```python
from build123d import *

# Parameters (mm, degrees)
SKETCH1_W           = 220
SKETCH1_H           = 220
BOSS_EXTRUDE1_DEPTH = 3
SKETCH2_W           = 220
SKETCH2_H           = 220
SKETCH2_W_2         = 204
SKETCH2_H_2         = 204
BOSS_EXTRUDE3_DEPTH = 22
SKETCH3_R           = 1
CUT_EXTRUDE1_DEPTH  = 313.1297807


with BuildPart() as part:
    # Sketch1 → Boss-Extrude1 (new body)
    with BuildSketch(Plane.XY):
        with Locations((110, 110)):
            Rectangle(SKETCH1_W, SKETCH1_H)
    extrude(amount=BOSS_EXTRUDE1_DEPTH)

    # Sketch2 → Boss-Extrude3 (add)
    with BuildSketch(Plane.XY.offset(3)):
        with Locations((110, 110)):
            Rectangle(SKETCH2_W, SKETCH2_H)
        with Locations((110, 110)):
            Rectangle(SKETCH2_W_2, SKETCH2_H_2, mode=Mode.SUBTRACT)
    extrude(amount=BOSS_EXTRUDE3_DEPTH)

    # Sketch3 → Cut-Extrude1 (cut, through all)
    with BuildSketch(Plane.XY.offset(25)):
        with Locations((4, 216)):
            Circle(SKETCH3_R)
        with Locations((110, 216)):
            Circle(SKETCH3_R)
        with Locations((216, 216)):
            Circle(SKETCH3_R)
        with Locations((216, 110)):
            Circle(SKETCH3_R)
        with Locations((216, 4)):
            Circle(SKETCH3_R)
        with Locations((110, 4)):
            Circle(SKETCH3_R)
        with Locations((4, 4)):
            Circle(SKETCH3_R)
        with Locations((4, 110)):
            Circle(SKETCH3_R)
    extrude(amount=-CUT_EXTRUDE1_DEPTH, mode=Mode.SUBTRACT)


solid = part.part
```
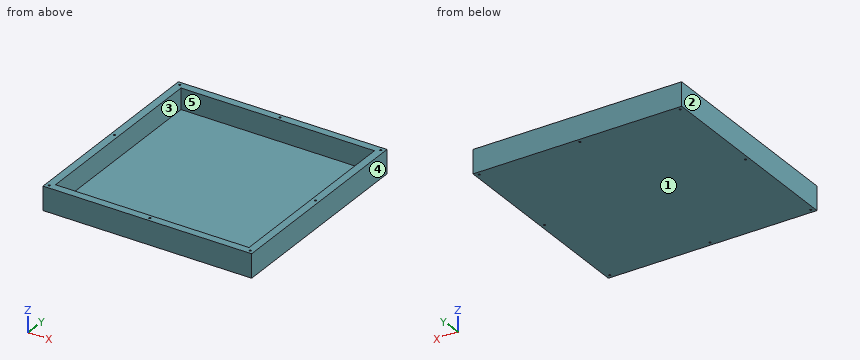
Geometry: final body of the model. Coordinates: model frame, mm. Face numbers are marked on the shaded views. A direction names the side the tool comes from. Give positions to 0.01 mm unless a question says otherwise; leave off trailing zeros. Write each loop counter-clockwise with the first axis right and the second up, starting at its lowest first coordinate (ties: lowest second). Pieces come first, ordered by that corner, then holes.
1. Line query: probe 1 along Y at (x, z) = (4, 5.5); probe 2 along Y at (x, z) = (110, 14). Output: solid intervals per line, ascending.
2. Pin query (flat end, axial travel): P1, Ø1.6, axis at x = 110, y = 4, coming from the +Z side; P2, Ø4, axis at x = 128, y = 181.5, coming from the +Z side. Return the tip coordinate at first contact, or that it passes through.
3. Section query A-A, the plane z = 7.5. Count the separate pieces of the cut face and the enclosed holes in it, then the cut area to 3 significant figures.
4. Reachability of the marked faces 4 and 5 from +Z, -Z, +X, -X, +Y, -Y: full face, straight path, thin tool, end or side. Return the list, or none.
5. Draft query along X for the marked faces 1, 2 and 3. Return one class per face: released by +X, released by -X, zero draft, split by the parting line, or undercut.
6. Section query B-B, the plane x = 201. Return loops of the section in (y, z).
Computed:
1. probe 1: y = 0 to 3, 5 to 109, 111 to 215, 217 to 220
1. probe 2: y = 0 to 3, 5 to 8, 212 to 215, 217 to 220
2. P1: passes through
2. P2: stops at z = 3
3. separate pieces: 1
3. enclosed holes: 9
3. area: 6,760 mm2
4. face 4: +Z, -Z, +X, +Y, -Y
4. face 5: +Z
5. face 1: zero draft
5. face 2: released by -X
5. face 3: undercut
6. outline: (0, 0) - (220, 0) - (220, 25) - (212, 25) - (212, 3) - (8, 3) - (8, 25) - (0, 25) - close
